from build123d import *

# Parameters (mm, degrees)
SKETCH_1_W                = 42
SKETCH_1_H                = 250
EXTRUDE_1_DEPTH           = 10
SKETCH_10_W               = 24
SKETCH_10_H               = 1
CUT_EXTRUDE_1_DEPTH       = 252.079668631
HOLE_WIZARD_M4_1_D        = 3.3
PATTERN_LINEAR_1_COUNT    = 6
PATTERN_LINEAR_1_PITCH    = 40
HOLE_WIZARD_M5_1_D        = 4.2
HOLE_WIZARD_1_D           = 4.5
HOLE_WIZARD_1_CBORE_D     = 8
HOLE_WIZARD_1_CBORE_DEPTH = 4.6
HOLE_WIZARD_M5_2_D        = 4.2
HOLE_WIZARD_M5_2_DEPTH    = 12.4
HOLE_WIZARD_M5_2_TIP      = 1.2618073


with BuildPart() as part:
    # 草图1 → 凸台-拉伸1 (new body)
    with BuildSketch(Plane(origin=(0, 0, 0), x_dir=(1, 0, 0), z_dir=(0, 1, 0))):
        Rectangle(SKETCH_1_W, SKETCH_1_H)
    extrude(amount=EXTRUDE_1_DEPTH)

    # 草图10 → 切除-拉伸1 (cut, through all)
    with BuildSketch(Plane(origin=(0, 0, -125), x_dir=(-1, 0, 0), z_dir=(0, 0, -1))):
        with Locations((0, 9.5)):
            Rectangle(SKETCH_10_W, SKETCH_10_H)
    extrude(amount=-CUT_EXTRUDE_1_DEPTH, mode=Mode.SUBTRACT)

    # M4 螺纹孔1 (through all)
    with Locations(Plane(origin=(-1.725383056, 9, -76.289623168), x_dir=(1, 0, 0), z_dir=(0, 1, 0))):
        with Locations((1.725383056, 31.710376832)):
            hole_wizard_m4_1 = Hole(HOLE_WIZARD_M4_1_D / 2)

    # 阵列(线性)1: M4 螺纹孔1 ×6
    with Locations(*[(0, 0, i * PATTERN_LINEAR_1_PITCH) for i in range(1, PATTERN_LINEAR_1_COUNT)]):
        add(hole_wizard_m4_1, mode=Mode.SUBTRACT)

    # M5 螺纹孔1 (through all)
    with Locations(Plane(origin=(0, 0, 0), x_dir=(-1, 0, 0), z_dir=(0, -1, 0))):
        with Locations((0, 55), (0, 115), (0, 85)):
            Hole(HOLE_WIZARD_M5_1_D / 2)

    # 打孔尺寸根据内六角圆柱头螺钉的类型1 (through all)
    with Locations(Plane(origin=(0, 0, 0), x_dir=(-1, 0, 0), z_dir=(0, -1, 0))):
        with Locations((16, -120), (16, -70), (-16, -70), (-16, -120)):
            CounterBoreHole(HOLE_WIZARD_1_D / 2, HOLE_WIZARD_1_CBORE_D / 2, HOLE_WIZARD_1_CBORE_DEPTH)

    # M5 螺纹孔2
    with Locations(Plane(origin=(0, 0, -125), x_dir=(-1, 0, 0), z_dir=(0, 0, -1))):
        with Locations((-15, 5), (15, 5)):
            Hole(HOLE_WIZARD_M5_2_D / 2, depth=HOLE_WIZARD_M5_2_DEPTH)
            with Locations((0, 0, -(HOLE_WIZARD_M5_2_DEPTH + HOLE_WIZARD_M5_2_TIP / 2))):  # 118° drill point
                Cone(0, HOLE_WIZARD_M5_2_D / 2, HOLE_WIZARD_M5_2_TIP, mode=Mode.SUBTRACT)


solid = part.part
Could you check a few things on this model? Use its own coordinates, in mm. A direction names the side the tool comes from. Coordinates: 2 decimals unless noted, no trailing zeros. Loops run counter-clockwise (first coordinate to the right, second up) from the corner with the lowest first, then second, coordinate; pieces in that order, holes last. Notation, with made-up numbers: (87, 7) -> (124, 7) arc R16 cw to (124, 13) -> close; hole circle Ø9 at (61.25, 12). An arc over 180 degrees is marked (long way). Answer in a Markdown table with one row per item.
(1) Imagine slicing it at C-C (z = 77). List the corners of the cut face in (x, y) for me, plus the area to 3 significant figures.
Results found:
| item | result |
|---|---|
| outline | (-21, 0) -> (21, 0) -> (21, 10) -> (12, 10) -> (12, 9) -> (-12, 9) -> (-12, 10) -> (-21, 10) -> close |
| area | 396 mm^2 |
(2) Thinking about a two-plate mould opening in Y: for faces 4 (the face through (16.867, 2.268, 73.905)), 5 (the face through (-18, 4.6, 122)), 6 (the face through (-15.273, 7.082, -118.713)), which applies, released by +Y, released by -Y, zero draft, split by the parting line, or undercut?
Results found:
| item | result |
|---|---|
| face 4 | zero draft |
| face 5 | released by -Y |
| face 6 | undercut |
(3) Will these pins go through, and if not, where does the flat tip stop? pin 1 Ø4 at (x, z) = (0, 12) entering from +Y; pin 2 Ø2.5 at (x, z) = (17.5, 69.5) entering from -Y; pin 3 Ø4 at (x, z) = (16, 120) entering from +Y.
Results found:
| item | result |
|---|---|
| pin 1 | stops at y = 9 |
| pin 2 | stops at y = 4.6 |
| pin 3 | passes through |
(4) If I drill on probe 1 along X at (y, z) = (6.75, 120); probe 2 along X at (y, z) = (5, -115); probe 3 along X at (y, z) = (5.75, -108), over which ranges is the centre line in solid material (lowest first)?
Results found:
| item | result |
|---|---|
| probe 1 | x = -21 to -18.25, -13.75 to 13.75, 18.25 to 21 |
| probe 2 | x = -21 to -17.1, -12.9 to -2.1, 2.1 to 12.9, 17.1 to 21 |
| probe 3 | x = -21 to -1.65, 1.65 to 21 |
(5) Imagine slicing it at B-B (z = -55). List the corners of the cut face in (x, y) for me, plus the area to 3 significant figures.
Results found:
| item | result |
|---|---|
| outline | (-21, 0) -> (-2.1, 0) -> (-2.1, 9) -> (-12, 9) -> (-12, 10) -> (-21, 10) -> close; (2.1, 0) -> (21, 0) -> (21, 10) -> (12, 10) -> (12, 9) -> (2.1, 9) -> close |
| area | 358 mm^2 |
(6) Imagine slicing it at A-A (z = -115). List the corners of the cut face in (x, y) for me, plus the area to 3 significant figures.
Results found:
| item | result |
|---|---|
| outline | (-21, 0) -> (-2.1, 0) -> (-2.1, 9) -> (-12, 9) -> (-12, 10) -> (-21, 10) -> close; (2.1, 0) -> (21, 0) -> (21, 10) -> (12, 10) -> (12, 9) -> (2.1, 9) -> close; hole circle Ø4.2 at (-15, 5); hole circle Ø4.2 at (15, 5) |
| area | 330 mm^2 |
(7) For faces 1 (the face through (14.727, 7.082, -118.713)), 2 (the face through (16, 10, -2)), 3 (the face through (14, 4.6, 72)), which set-ups out of +Z, -Z, +X, -X, +Y, -Y let a thin tool reach every point of the face, with its end or its side?
Results found:
| item | result |
|---|---|
| face 1 | -Z |
| face 2 | +Z, -Z, +X, -X, +Y |
| face 3 | -Y |
